The listing builds one solid part. Answer for the finished solid, in the listing's coordinates (mm). A direction names the side the tool comes from. Give positions to 0.01 mm unless a question says otherwise; leave off trailing zeros. Order: outer loops, then holes, each group sorted by start corner. A loop starts at its lowest first (then second) coordinate and runs counter-clockwise, first axis right, second up.
```python
from build123d import *
from build123d.topology import SkipClean

# Parameters (mm, degrees)
SKETCH2_W            = 35
SKETCH2_H            = 55
BOSS_EXTRUDE1_DEPTH  = 45
BOSS_EXTRUDE2_DEPTH  = 5
SKETCH6_R            = 17.5
BOSS_EXTRUDE3_DEPTH  = 12
BOSS_EXTRUDE4_START  = 5
BOSS_EXTRUDE4_DEPTH  = 5
BOSS_EXTRUDE5_START  = 12
SKETCH8_R            = 17.5
BOSS_EXTRUDE5_DEPTH  = 12
BOSS_EXTRUDE6_START  = -12
BOSS_EXTRUDE6_DEPTH  = 12
BOSS_EXTRUDE7_DEPTH  = 12
SKETCH14_W           = 24.5
SKETCH14_H           = 45.4
SKETCH14_R           = 2.449946242
CUT_EXTRUDE3_DEPTH   = 12
SKETCH15_R           = 21.1
CUT_EXTRUDE4_DEPTH   = 12
CUT_EXTRUDE5_DEPTH   = 139.069755203
SKETCH21_R           = 1.25
CUT_EXTRUDE7_DEPTH   = 12
SKETCH23_R           = 10.1
BOSS_EXTRUDE8_DEPTH  = 6
SKETCH24_R           = 8.5
CUT_EXTRUDE8_DEPTH   = 6
SKETCH25_R           = 2.7
CUT_EXTRUDE9_DEPTH   = 18
BOSS_EXTRUDE9_START  = -12
BOSS_EXTRUDE9_DEPTH  = 12
SKETCH30_R           = 1.25
CUT_EXTRUDE11_DEPTH  = 12
SKETCH31_R           = 2
CUT_EXTRUDE12_DEPTH  = 2.5
BOSS_EXTRUDE11_DEPTH = 12
SKETCH33_W           = 17.5
SKETCH33_H           = 5.5
SKETCH33_W_2         = 45
SKETCH33_H_2         = 11
CUT_EXTRUDE13_DEPTH  = 40


with BuildPart() as part:
    # Sketch2 → Boss-Extrude1 (new body)
    with BuildSketch(Plane.XY):
        with BuildLine():
            ThreePointArc((-17.5, 27.5), (0, 45), (17.5, 27.5))
            Line((17.5, 27.5), (-17.5, 27.5))
        make_face()
        Rectangle(SKETCH2_W, SKETCH2_H)
        with BuildLine():
            ThreePointArc((17.5, -27.5), (0, -45), (-17.5, -27.5))
            Line((-17.5, -27.5), (17.5, -27.5))
        make_face()
    extrude(amount=BOSS_EXTRUDE1_DEPTH)

    # Sketch5 → Boss-Extrude2 (add)
    with SkipClean():  # the faces are left unmerged after this step: merging them gives an invalid solid
        with BuildSketch(Plane.XY.offset(45)):
            with BuildLine():
                ThreePointArc((17.5, 27.5), (0, 45), (-17.5, 27.5))
                ThreePointArc((-17.5, 27.5), (0, 10), (17.5, 27.5))
            make_face()
        extrude(amount=BOSS_EXTRUDE2_DEPTH)

    # Sketch6 → Boss-Extrude3 (add)
    with BuildSketch(Plane.XY.offset(50)):
        with BuildLine():
            Line((-17.5, 67.5), (17.5, 67.5))
            ThreePointArc((17.5, 67.5), (0, 85), (-17.5, 67.5))
        make_face()
        with BuildLine():
            Line((17.5, 27.5), (17.5, 67.5))
            Line((17.5, 67.5), (-17.5, 67.5))
            Line((-17.5, 67.5), (-17.5, 27.5))
            ThreePointArc((-17.5, 27.5), (0, 45), (17.5, 27.5))
        make_face()
        with Locations(Location((0, 27.5, 0), (0, 0, 180))):
            Circle(SKETCH6_R)
    extrude(amount=BOSS_EXTRUDE3_DEPTH)

    # Sketch7 → Boss-Extrude4 (add)
    with SkipClean():  # the faces are left unmerged after this step: merging them gives an invalid solid
        with BuildSketch(Plane(origin=(0, 0, 0), x_dir=(-1, 0, 0), z_dir=(0, 0, -1)).offset(BOSS_EXTRUDE4_START)):
            with BuildLine():
                ThreePointArc((17.5, 27.5), (0, 10), (-17.5, 27.5))
                ThreePointArc((-17.5, 27.5), (0, 45), (17.5, 27.5))
            make_face()
        extrude(amount=-BOSS_EXTRUDE4_DEPTH)
    add(part.part.scale(1), mode=Mode.REPLACE)  # the faces are merged on a copy

    # Sketch8 → Boss-Extrude5 (add)
    with SkipClean():  # the faces are left unmerged after this step: merging them gives an invalid solid
        with BuildSketch(Plane(origin=(0, 0, -5), x_dir=(-1, 0, 0), z_dir=(0, 0, -1)).offset(BOSS_EXTRUDE5_START)):
            with BuildLine():
                Line((17.5, 67.5), (-17.5, 67.5))
                ThreePointArc((-17.5, 67.5), (0, 85), (17.5, 67.5))
            make_face()
            with BuildLine():
                ThreePointArc((-17.5, 27.5), (0, 45), (17.5, 27.5))
                Line((17.5, 27.5), (17.5, 67.5))
                Line((17.5, 67.5), (-17.5, 67.5))
                Line((-17.5, 67.5), (-17.5, 27.5))
            make_face()
            with Locations((0, 27.5)):
                Circle(SKETCH8_R)
        extrude(amount=-BOSS_EXTRUDE5_DEPTH)

    # Sketch11 → Boss-Extrude6 (add)
    with BuildSketch(Plane.XY.offset(62).offset(BOSS_EXTRUDE6_START)):
        with BuildLine():
            Line((-17.5, 67.5), (-17.5, 27.5))
            ThreePointArc((-17.5, 27.5), (0, 10), (17.5, 27.5))
            Line((17.5, 27.5), (17.5, 67.5))
            ThreePointArc((17.5, 67.5), (0, 115.060885195), (-17.5, 67.5))
        make_face()
    extrude(amount=BOSS_EXTRUDE6_DEPTH)

    # Sketch12 → Boss-Extrude7 (add)
    with BuildSketch(Plane(origin=(0, 0, -17), x_dir=(-1, 0, 0), z_dir=(0, 0, -1))):
        with BuildLine():
            ThreePointArc((17.5, 67.5), (0, 115.060885195), (-17.5, 67.5))
            ThreePointArc((-17.5, 67.5), (0, 85), (17.5, 67.5))
        make_face()
    extrude(amount=-BOSS_EXTRUDE7_DEPTH)

    # Sketch14 → Cut-Extrude3 (cut)
    # profile 1 of 2: a face of its own
    with BuildSketch(Plane.XY.offset(62)):
        with Locations((0, 77.710885195)):
            Rectangle(SKETCH14_W, SKETCH14_H)
        with Locations((0, 88.060885195)):
            Circle(SKETCH14_R, mode=Mode.SUBTRACT)
    # profile 2 of 2: a face of its own
    with BuildSketch(Plane.XY.offset(62)):
        with Locations((0, 88.060885195)):
            Circle(SKETCH14_R)
    extrude(amount=-CUT_EXTRUDE3_DEPTH, mode=Mode.SUBTRACT)

    # Sketch15 → Cut-Extrude4 (cut)
    with BuildSketch(Plane(origin=(0, 0, -17), x_dir=(-1, 0, 0), z_dir=(0, 0, -1))):
        with Locations((0, 88.060885195)):
            Circle(SKETCH15_R)
    extrude(amount=-CUT_EXTRUDE4_DEPTH, mode=Mode.SUBTRACT)

    # Sketch17 → Cut-Extrude5 (cut, through all)
    with BuildSketch(Plane.ZY.offset(17.5)):
        Polygon((10, -27.5), (22.5, -27.5), (35, -27.5), (35, -15.5), (10, -15.5), align=None)
        Polygon((35, -27.5), (22.5, -27.5), (10, -27.5), (10, -45), (35, -45), align=None)
    extrude(amount=-CUT_EXTRUDE5_DEPTH, mode=Mode.SUBTRACT)

    # Sketch21 → Cut-Extrude7 (cut)
    with BuildSketch(Plane.XY.offset(45)):
        with Locations((8, -27.5)):
            Circle(SKETCH21_R)
        with Locations((5.656854249, -33.156854249)):
            Circle(SKETCH21_R)
        with Locations((0, -35.5)):
            Circle(SKETCH21_R)
        with Locations((-5.656854249, -33.156854249)):
            Circle(SKETCH21_R)
        with Locations((-8, -27.5)):
            Circle(SKETCH21_R)
        with Locations((-5.656854249, -21.843145751)):
            Circle(SKETCH21_R)
        with Locations((0, -19.5)):
            Circle(SKETCH21_R)
        with Locations((5.656854249, -21.843145751)):
            Circle(SKETCH21_R)
    extrude(amount=-CUT_EXTRUDE7_DEPTH, mode=Mode.SUBTRACT)

    # Sketch23 → Boss-Extrude8 (add)
    with BuildSketch(Plane(origin=(0, 0, 0), x_dir=(-1, 0, 0), z_dir=(0, 0, -1))):
        with Locations(Location((0, -27.5, 0), (0, 0, 180))):
            Circle(SKETCH23_R)
    extrude(amount=BOSS_EXTRUDE8_DEPTH)

    # Sketch24 → Cut-Extrude8 (cut)
    with BuildSketch(Plane(origin=(0, 0, -6), x_dir=(-1, 0, 0), z_dir=(0, 0, -1))):
        with Locations((0, -27.5)):
            Circle(SKETCH24_R)
    extrude(amount=-CUT_EXTRUDE8_DEPTH, mode=Mode.SUBTRACT)

    # Sketch25 → Cut-Extrude9 (cut)
    with BuildSketch(Plane(origin=(0, 0, 0), x_dir=(-1, 0, 0), z_dir=(0, 0, -1))):
        with Locations((0, -27.5)):
            Circle(SKETCH25_R)
    extrude(amount=-CUT_EXTRUDE9_DEPTH, mode=Mode.SUBTRACT)

    # Sketch26 → Boss-Extrude9 (add)
    with BuildSketch(Plane.XY.offset(62).offset(BOSS_EXTRUDE9_START)):
        with BuildLine():
            ThreePointArc((-17.5, 67.5), (-23.313699367, 74.442095901), (-26.505269682, 82.915918813))
            ThreePointArc((-26.505269682, 82.915918813), (-22.976087169, 55.049770191), (-17.5, 27.5))
            Line((-17.5, 27.5), (-17.5, 67.5))
        make_face()
        with BuildLine():
            ThreePointArc((17.5, 27.5), (22.976087169, 55.049770191), (26.505269682, 82.915918813))
            ThreePointArc((26.505269682, 82.915918813), (23.313699367, 74.442095901), (17.5, 67.5))
            Line((17.5, 67.5), (17.5, 27.5))
        make_face()
    extrude(amount=BOSS_EXTRUDE9_DEPTH)

    # Sketch30 → Cut-Extrude11 (cut)
    with BuildSketch(Plane.XY.offset(62)):
        with Locations((15, 92.910885195)):
            Circle(SKETCH30_R)
        with Locations((15, 75.910885195)):
            Circle(SKETCH30_R)
        with Locations((15, 58.910885195)):
            Circle(SKETCH30_R)
        with Locations(Location((-15, 92.910885195, 0), (0, 0, 180))):
            Circle(SKETCH30_R)
        with Locations(Location((-15, 75.910885195, 0), (0, 0, 180))):
            Circle(SKETCH30_R)
        with Locations(Location((-15, 58.910885195, 0), (0, 0, 180))):
            Circle(SKETCH30_R)
    extrude(amount=-CUT_EXTRUDE11_DEPTH, mode=Mode.SUBTRACT)

    # Sketch31 → Cut-Extrude12 (cut)
    with BuildSketch(Plane(origin=(0, 0, 50), x_dir=(-1, 0, 0), z_dir=(0, 0, -1))):
        with Locations((15, 92.910885195)):
            Circle(SKETCH31_R)
        with Locations((15, 75.910885195)):
            Circle(SKETCH31_R)
        with Locations((15, 58.910885195)):
            Circle(SKETCH31_R)
        with Locations(Location((-15, 58.910885195, 0), (0, 0, 180))):
            Circle(SKETCH31_R)
        with Locations(Location((-15, 75.910885195, 0), (0, 0, 180))):
            Circle(SKETCH31_R)
        with Locations(Location((-15, 92.910885195, 0), (0, 0, 180))):
            Circle(SKETCH31_R)
    extrude(amount=-CUT_EXTRUDE12_DEPTH, mode=Mode.SUBTRACT)

    # Sketch32 → Boss-Extrude11 (add)
    with BuildSketch(Plane(origin=(0, 0, -17), x_dir=(-1, 0, 0), z_dir=(0, 0, -1))):
        with BuildLine():
            ThreePointArc((-17.5, 67.5), (-23.313699367, 74.442095901), (-26.505269682, 82.915918813))
            ThreePointArc((-26.505269682, 82.915918813), (-22.976087169, 55.049770191), (-17.5, 27.5))
            Line((-17.5, 27.5), (-17.5, 67.5))
        make_face()
        with BuildLine():
            ThreePointArc((17.5, 27.5), (22.976087169, 55.049770191), (26.505269682, 82.915918813))
            ThreePointArc((26.505269682, 82.915918813), (23.313699367, 74.442095901), (17.5, 67.5))
            Line((17.5, 67.5), (17.5, 27.5))
        make_face()
    extrude(amount=-BOSS_EXTRUDE11_DEPTH)

    # Sketch33 → Cut-Extrude13 (cut)
    with BuildSketch(Plane.ZY.offset(17.5)):
        with Locations((13.75, 31.25)):
            Rectangle(SKETCH33_W, SKETCH33_H)
        with Locations((31.25, 31.25)):
            Rectangle(SKETCH33_W, SKETCH33_H)
        with Locations((22.5, 39.5)):
            Rectangle(SKETCH33_W_2, SKETCH33_H_2)
    extrude(amount=-CUT_EXTRUDE13_DEPTH, mode=Mode.SUBTRACT)


solid = part.part
```
1) Find section B-B (z = 18). Write down the section's boundary in (x, y), then the cut area to 3 significant figures.
Geometry says:
outline: (-17.5, -15.5) - (17.5, -15.5) - (17.5, 27.5) arc R17.5 ccw to (17.47, 28.5) - (-17.47, 28.5) arc R17.5 ccw to (-17.5, 27.5) - close
area: 1,540 mm2
2) Find section D-D (y = -14). Write down the section's boundary in (x, z).
Geometry says:
outline: (-17.5, 0) - (17.5, 0) - (17.5, 45) - (-17.5, 45) - close
3) Given P1, Ø6.5, axis at x = 15, y = 92.91, coming from the -Z side; P2, Ø1.5, axis at x = 0, y = -19.5, coming from the -Z side; P3, Ø5, axis at x = 18, z = 43, coming from the +Y side, each flat-ended and moving along its own axis, determine where each tip first touches the part or whether it passes through.
Geometry says:
P1: stops at z = 50
P2: stops at z = -6
P3: stops at y = 34
4) Find section C-C (z = 38). Count the separate pieces of the cut face and the enclosed holes in it, then the cut area to 3 significant figures.
Geometry says:
separate pieces: 1
enclosed holes: 8
area: 2,400 mm2
5) Find section A-A (y = 32). Write down the section's boundary in (x, z), then the cut area to 3 significant figures.
Geometry says:
outline: (-18.53, -17) - (18.53, -17) - (18.53, -5) - (16.91, -5) - (16.91, 5) - (-16.91, 5) - (-16.91, -5) - (-18.53, -5) - close; (-18.53, 50) - (-16.91, 50) - (-16.91, 40) - (16.91, 40) - (16.91, 50) - (18.53, 50) - (18.53, 62) - (-18.53, 62) - close
area: 1,570 mm2
6) For a pull along Z with two mould halves and no side action, classify faces 6 (the flat face through (0, -16, 45)), 7 (the flat face through (12.25, 77, 56)), 8 (the flat face through (0, 31, 5)) as +Z half, -Z half, draft (parallel to the pull), parting line (faces both ways), or undercut.
Geometry says:
face 6: +Z half
face 7: draft
face 8: undercut
7) A tool of negligible diameter and unlimited length cuts with its end or side. For faces 1 (the cylindrical face through (0.351, -24.823, 4.93)), 2 (the cylindrical face through (-14.566, 73.958, 51.232)), 3 (the flat face through (0, -15.5, 23)), 4 (the flat face through (0, 34, 42)), 5 (the flat face through (0, 100.411, 56)), from which of +Z, -Z, +X, -X, +Y, -Y can it reach the whole face along a straight path? Write none if from no direction.
Geometry says:
face 1: -Z
face 2: none
face 3: +X, -X, -Y
face 4: +X, -X, +Y
face 5: +Z, -Z
8) Straight lines are drawn through the part: probe 1 along Y at (x, z) = (0, -3); probe 2 along Z at (x, y) = (19, 100.5); probe 3 along Y at (x, z) = (-1, 57.5). For each, find the intervals that lie inside material, in ascending order.
Geometry says:
probe 1: y = -37.6 to -36, -19 to -17.4, 10 to 45
probe 2: z = -17 to -5, 50 to 62
probe 3: y = 10.03 to 55.01, 100.41 to 115.04
